from build123d import *

# Parameters (mm, degrees)
SKETCH1_W                        = 85.09
SKETCH1_H                        = 68.58
BOSS_EXTRUDE1_DEPTH              = 48.26
SKETCH2_W                        = 72.39
SKETCH2_H                        = 55.88
CUT_EXTRUDE1_DEPTH               = 25.4
SKETCH4_W                        = 55.88
SKETCH4_H                        = 21.59
SKETCH4_H_2                      = 15.24
CUT_EXTRUDE2_DEPTH               = 86.09
SKETCH5_W                        = 81.28
SKETCH5_H                        = 55.88
CUT_EXTRUDE4_DEPTH               = 20.32
F_30_0_1285_DIAMETER_HOLE1_D     = 3.2639
F_30_0_1285_DIAMETER_HOLE1_DEPTH = 12.7
F_30_0_1285_DIAMETER_HOLE1_TIP   = 0.980574487
SKETCH9_W                        = 33.02
SKETCH9_H                        = 16.51
SKETCH9_H_2                      = 20.32
CUT_EXTRUDE5_DEPTH               = 69.58
SKETCH10_R                       = 3.175
SKETCH10_R_2                     = 1.63195
BOSS_EXTRUDE2_DEPTH              = 2.54
CUT_EXTRUDE6_REACH               = 24.86
SKETCH10_3_R                     = 1.63195
SKETCH12_W                       = 6.35
SKETCH12_H                       = 2.54
BOSS_EXTRUDE3_DEPTH              = 22.606
SKETCH13_W                       = 6.35
SKETCH13_H                       = 2.54
BOSS_EXTRUDE4_DEPTH              = 33.782


with BuildPart() as part:
    # Sketch1 → Boss-Extrude1 (new body)
    with BuildSketch(Plane(origin=(0, 0, 0), x_dir=(1, 0, 0), z_dir=(0, 1, 0))):
        with Locations((42.545, 34.29)):
            Rectangle(SKETCH1_W, SKETCH1_H)
    extrude(amount=BOSS_EXTRUDE1_DEPTH)

    # Sketch2 → Cut-Extrude1 (cut)
    with BuildSketch(Plane(origin=(0, 48.26, 0), x_dir=(1, 0, 0), z_dir=(0, 1, 0))):
        with Locations((42.545, 34.29)):
            Rectangle(SKETCH2_W, SKETCH2_H)
    extrude(amount=-CUT_EXTRUDE1_DEPTH, mode=Mode.SUBTRACT)

    # Sketch4 → Cut-Extrude2 (cut, through all)
    with BuildSketch(Plane.ZY):
        with Locations((-34.29, 33.655)):
            Rectangle(SKETCH4_W, SKETCH4_H)
        with Locations((-34.29, 12.7)):
            Rectangle(SKETCH4_W, SKETCH4_H_2)
    extrude(amount=-CUT_EXTRUDE2_DEPTH, mode=Mode.SUBTRACT)

    # Sketch5 → Cut-Extrude4 (cut)
    with BuildSketch(Plane(origin=(0, 0, 0), x_dir=(-1, 0, 0), z_dir=(0, -1, 0))):
        with Locations((-42.545, 34.29)):
            Rectangle(SKETCH5_W, SKETCH5_H)
    extrude(amount=-CUT_EXTRUDE4_DEPTH, mode=Mode.SUBTRACT)

    # 30 _0.1285_ Diameter Hole1
    with Locations(Plane(origin=(22.86, 48.26, -3.175), x_dir=(0, 0, 1), z_dir=(0, 1, 0))):
        with Locations((0, 0), (-62.23, 0), (-62.23, 39.37), (0, 39.37)):
            Hole(F_30_0_1285_DIAMETER_HOLE1_D / 2, depth=F_30_0_1285_DIAMETER_HOLE1_DEPTH)
            with Locations((0, 0, -(F_30_0_1285_DIAMETER_HOLE1_DEPTH + F_30_0_1285_DIAMETER_HOLE1_TIP / 2))):  # 118° drill point
                Cone(0, F_30_0_1285_DIAMETER_HOLE1_D / 2, F_30_0_1285_DIAMETER_HOLE1_TIP, mode=Mode.SUBTRACT)

    # Sketch9 → Cut-Extrude5 (cut, through all)
    with BuildSketch(Plane.XY):
        with Locations((22.86, 12.065)):
            Rectangle(SKETCH9_W, SKETCH9_H)
        with Locations((22.86, 33.02)):
            Rectangle(SKETCH9_W, SKETCH9_H_2)
        with Locations((62.23, 33.02)):
            Rectangle(SKETCH9_W, SKETCH9_H_2)
        with Locations((62.23, 12.065)):
            Rectangle(SKETCH9_W, SKETCH9_H)
    extrude(amount=-CUT_EXTRUDE5_DEPTH, mode=Mode.SUBTRACT)

    # Sketch10 → Boss-Extrude2 (add)
    with BuildSketch(Plane(origin=(0, 22.86, 0), x_dir=(1, 0, 0), z_dir=(0, 1, 0))):
        with Locations((57.15, 58.42)):
            Circle(SKETCH10_R)
        with Locations((57.15, 58.42)):
            Circle(SKETCH10_R_2, mode=Mode.SUBTRACT)
        with Locations((55.88, 10.16)):
            Circle(SKETCH10_R)
        with Locations((55.88, 10.16)):
            Circle(SKETCH10_R_2, mode=Mode.SUBTRACT)
        with Locations((5.08, 25.4)):
            Circle(SKETCH10_R)
        with Locations((5.08, 25.4)):
            Circle(SKETCH10_R_2, mode=Mode.SUBTRACT)
        with Locations((5.08, 53.34)):
            Circle(SKETCH10_R)
        with Locations((5.08, 53.34)):
            Circle(SKETCH10_R_2, mode=Mode.SUBTRACT)
    extrude(amount=BOSS_EXTRUDE2_DEPTH)

    # Sketch10_3 → Cut-Extrude6 (cut, up to next)
    with BuildSketch(Plane(origin=(0, 22.86, 0), x_dir=(1, 0, 0), z_dir=(0, 1, 0)), mode=Mode.PRIVATE) as cut_extrude6_sk1:
        with Locations((57.15, 58.42)):
            Circle(SKETCH10_3_R)
    cut_extrude6_tool1 = extrude(cut_extrude6_sk1.sketch, amount=-CUT_EXTRUDE6_REACH, mode=Mode.PRIVATE) & part.part
    add(cut_extrude6_tool1.solids().sort_by_distance((57.15, 22.86, -58.42))[0], mode=Mode.SUBTRACT)
    # Sketch10_3 → Cut-Extrude6 (cut, up to next)
    with BuildSketch(Plane(origin=(0, 22.86, 0), x_dir=(1, 0, 0), z_dir=(0, 1, 0)), mode=Mode.PRIVATE) as cut_extrude6_sk2:
        with Locations((55.88, 10.16)):
            Circle(SKETCH10_3_R)
    cut_extrude6_tool2 = extrude(cut_extrude6_sk2.sketch, amount=-CUT_EXTRUDE6_REACH, mode=Mode.PRIVATE) & part.part
    add(cut_extrude6_tool2.solids().sort_by_distance((55.88, 22.86, -10.16))[0], mode=Mode.SUBTRACT)
    # Sketch10_3 → Cut-Extrude6 (cut, up to next)
    with BuildSketch(Plane(origin=(0, 22.86, 0), x_dir=(1, 0, 0), z_dir=(0, 1, 0)), mode=Mode.PRIVATE) as cut_extrude6_sk3:
        with Locations((5.08, 25.4)):
            Circle(SKETCH10_3_R)
    cut_extrude6_tool3 = extrude(cut_extrude6_sk3.sketch, amount=-CUT_EXTRUDE6_REACH, mode=Mode.PRIVATE) & part.part
    add(cut_extrude6_tool3.solids().sort_by_distance((5.08, 22.86, -25.4))[0], mode=Mode.SUBTRACT)
    # Sketch10_3 → Cut-Extrude6 (cut, up to next)
    with BuildSketch(Plane(origin=(0, 22.86, 0), x_dir=(1, 0, 0), z_dir=(0, 1, 0)), mode=Mode.PRIVATE) as cut_extrude6_sk4:
        with Locations((5.08, 53.34)):
            Circle(SKETCH10_3_R)
    cut_extrude6_tool4 = extrude(cut_extrude6_sk4.sketch, amount=-CUT_EXTRUDE6_REACH, mode=Mode.PRIVATE) & part.part
    add(cut_extrude6_tool4.solids().sort_by_distance((5.08, 22.86, -53.34))[0], mode=Mode.SUBTRACT)

    # Sketch12 → Boss-Extrude3 (add)
    with BuildSketch(Plane(origin=(0, 22.86, 0), x_dir=(1, 0, 0), z_dir=(0, 1, 0))):
        with Locations((81.915, 30.96)):
            Rectangle(SKETCH12_W, SKETCH12_H)
    extrude(amount=BOSS_EXTRUDE3_DEPTH)

    # Sketch13 → Boss-Extrude4 (add)
    with BuildSketch(Plane(origin=(0, 0, -32.23), x_dir=(-1, 0, 0), z_dir=(0, 0, -1))):
        with Locations((-81.915, 34.29)):
            Rectangle(SKETCH13_W, SKETCH13_H)
    extrude(amount=BOSS_EXTRUDE4_DEPTH)


solid = part.part
Can you work these out from the model? Positions are in its coordinate system, mm. A direction names the side the tool comes from. Round coordinates to 2 decimals unless told otherwise and drop trailing zeros. Write each loop counter-clockwise with the first axis right and the second up, starting at its lowest first coordinate (ties: lowest second). Pieces come first, ordered by that corner, then holes. Notation, with made-up numbers: (62.5, -30) -> (97.5, -30) arc R19 cw to (97.5, 1) -> close; hole circle Ø4 at (71, -12.75). An arc over 180 degrees is marked (long way). One line per question, with ' | ' between items. Start each with the question number.
1) Suppose I cut it at A-A on x = 22.86. Write out the boundary of the cut face in (y, z), then the cut area to 3 significant figures.
2) I'm going to push flat-ended pins straight in: P1, Ø3, axis at x = 24.5, z = -52, coming from the -Y side; P2, Ø16.5, axis at x = 61, y = 14.5, coming from the +Z side; P3, Ø3, axis at x = 5.08, z = -53.34, coming from the -Y side. Where does each tip first touch, or does it pass through?
3) I need wall thicknesses on line 1 (Y direction, x = 77, z = -65.5); line 2 (X direction, y = 29.5, z = -63.5); line 3 (Y direction, x = 79.5, z = -34). Which ranges of each line are inside material? Lowest first, please. Write a range as [from, to].
4) Suppose I cut it at B-B on y = 31. Write out the boundary of the cut face in (x, z).
5) On a 3-axis mill with a long thin cutter (end or side, diameter ignored), from which of +Z, -Z, +X, -X, +Y, -Y can I reach the whole of each face in a straight line? I mean faces 3 (the cylindrical face through (63.848, 45.684, -2.963)), 4 (the cylindrical face through (4.67, 24.11, -56.49)), 5 (the flat face through (82, 33.02, -47)), 6 (the flat face through (39.37, 12, -3)), 7 (the flat face through (83.185, 3, -34)). Say none if no direction works.
6) Suppose I cut it at D-D on x = 5.08. Write out the boundary of the cut face in (y, z) (3 decimals), then the cut area to 3 significant figures.
7) Suppose I cut it at C-C on z = -53.34. Count the separate pieces of the cut face and the enclosed holes in it, then the cut area to 3 significant figures.
8) If we mould it in two halves opening along X, with no side actions, what happens to faces 1 (the flat face through (82, 28, -32.23)), 2 (the flat face through (6.35, 12, -65))? For each: released by +X, released by -X, zero draft, split by the parting line, or undercut.
Return value:
1) outline: (0, -68.58) -> (3.81, -68.58) -> (3.81, -62.23) -> (0, -62.23) -> close; (0, -6.35) -> (3.81, -6.35) -> (3.81, 0) -> (0, 0) -> close; (20.32, -68.58) -> (22.86, -68.58) -> (22.86, 0) -> (20.32, 0) -> close; (43.18, -68.58) -> (48.26, -68.58) -> (48.26, -67.04) -> (43.18, -67.04) -> close; (43.18, -63.77) -> (48.26, -63.77) -> (48.26, -62.23) -> (43.18, -62.23) -> close; (43.18, -6.35) -> (48.26, -6.35) -> (48.26, -4.81) -> (43.18, -4.81) -> close; (43.18, -1.54) -> (48.26, -1.54) -> (48.26, 0) -> (43.18, 0) -> close | area: 254 mm2
2) P1: stops at y = 20.32 | P2: stops at z = 0 | P3: stops at y = 44.45
3) line 1: y = [0, 3.81], [20.32, 22.86], [43.18, 48.26] | line 2: x = [0, 6.35], [39.37, 45.72], [78.74, 85.09] | line 3: y = [20.32, 22.86], [33.02, 35.56], [44.45, 48.26]
4) outline: (0, -68.58) -> (6.35, -68.58) -> (6.35, -62.23) -> (0, -62.23) -> close; (0, -6.35) -> (6.35, -6.35) -> (6.35, 0) -> (0, 0) -> close; (39.37, -68.58) -> (45.72, -68.58) -> (45.72, -62.23) -> (39.37, -62.23) -> close; (39.37, -6.35) -> (45.72, -6.35) -> (45.72, 0) -> (39.37, 0) -> close; (78.74, -68.58) -> (85.09, -68.58) -> (85.09, -62.23) -> (78.74, -62.23) -> close; (78.74, -32.23) -> (85.09, -32.23) -> (85.09, -29.69) -> (78.74, -29.69) -> close; (78.74, -6.35) -> (85.09, -6.35) -> (85.09, 0) -> (78.74, 0) -> close
5) face 3: +Y | face 4: none | face 5: +X, -X | face 6: +Z, -Z | face 7: -Y
6) outline: (0, -68.58) -> (48.26, -68.58) -> (48.26, 0) -> (0, 0) -> (0, -6.35) -> (20.32, -6.35) -> (20.32, -23.768) -> (25.4, -23.768) -> (25.4, -22.225) -> (22.86, -22.225) -> (22.86, -6.35) -> (44.45, -6.35) -> (44.45, -62.23) -> (22.86, -62.23) -> (22.86, -56.515) -> (25.4, -56.515) -> (25.4, -54.972) -> (20.32, -54.972) -> (20.32, -62.23) -> (0, -62.23) -> close; (20.32, -51.708) -> (25.4, -51.708) -> (25.4, -50.165) -> (22.86, -50.165) -> (22.86, -28.575) -> (25.4, -28.575) -> (25.4, -27.032) -> (20.32, -27.032) -> close | area: 967 mm2
7) separate pieces: 7 | enclosed holes: 0 | area: 300 mm2
8) face 1: zero draft | face 2: undercut
